Work out the finished part from the listing and answer in its coordinate system (mm). A direction names the side the tool comes from. Coordinates: 2 decimals unless noted, no trailing zeros. Loops run counter-clockwise (first coordinate to the right, second up) from the corner with the lowest first, then second, coordinate; pieces in that order, holes last. Notation, with made-up numbers: M 6.5,6 L 24.5,6 A35 ccw 24.5,41 Z; hole C 27.25,-30.75 d9. An arc over 180 degrees is marked long. Write each question's results on one line, items separated by ' | '.
```python
from build123d import *

# Parameters (mm, degrees)
EXTRUDE_THIN1_DEPTH = 80
BOSS_EXTRUDE1_REACH = 163.189
SKETCH2_W           = 20
SKETCH2_H           = 80


with BuildPart() as part:
    # Sketch1 → Extrude-Thin1 (new body)
    with BuildSketch(Plane.XY):
        with BuildLine():
            Line((0, 80), (0, 0))
            Line((0, 0), (85, 0))
            ThreePointArc((85, 0), (105.664665971, 60.876142901), (159.11809549, 96.592582629))
            Line((159.11809549, 96.592582629), (161.188647851, 88.865176019))
            ThreePointArc((161.188647851, 88.865176019), (109.643288684, 52.776567335), (93.348486101, -8))
            Line((93.348486101, -8), (-8, -8))
            Line((-8, -8), (-8, 80))
            Line((-8, 80), (0, 80))
        make_face()
    extrude(amount=EXTRUDE_THIN1_DEPTH)

    # Sketch2 → Boss-Extrude1 (add, up to next)
    with BuildSketch(Plane(origin=(0, 0, 0), x_dir=(0, 0, -1), z_dir=(1, 0, 0)), mode=Mode.PRIVATE) as boss_extrude1_sk1:
        with Locations((-40, 40)):
            Rectangle(SKETCH2_W, SKETCH2_H)
    boss_extrude1_tool1 = extrude(boss_extrude1_sk1.sketch, amount=BOSS_EXTRUDE1_REACH, mode=Mode.PRIVATE) - part.part
    add(boss_extrude1_tool1.solids().sort_by_distance((0, 40, 40))[0])


solid = part.part
```
1) Find section A-A, the plane z = 22.5. Give the vertices of the cut face in (x, y).
Check result:
outline: M -8,-8 L 93.35,-8 A92 cw 161.19,88.87 L 159.12,96.59 A100 ccw 85,0 L 0,0 L 0,80 L -8,80 Z
2) Given pin 1 Ø4 at (x, z) = (42, 55) entering from +Y; pin 2 Ø3 at (x, z) = (104, 61.5) entering from +Y; pin 3 Ø10 at (x, z) = (69.5, 30.5) entering from +Y, each flat-ended and moving along its own axis, determine where each tip first touches the part or whether it passes through.
Check result:
pin 1: y = 0 | pin 2: y = 60.66 | pin 3: y = 80
3) Straight lines are drawn through the part: probe 1 along X at (y, z) = (25, 10); probe 2 along X at (y, z) = (34, 60); probe 3 along Y at (x, z) = (83, 62). For each, find the intervals that lie inside material, in ascending order. Write a range as [from, to].
Check result:
probe 1: [-8, 0], [88.18, 96.46] | probe 2: [-8, 0], [90.96, 99.51] | probe 3: [-8, 0]
4) Find section B-B, the plane x = 66. Give the vertices of the cut face in (y, z).
Check result:
outline: M -8,0 L 0,0 L 0,30 L 80,30 L 80,50 L 0,50 L 0,80 L -8,80 Z
5) Find section C-C, the plane y = 16. Give the vertices of the cut face in (x, z), and give its area (3 significant figures).
Check result:
outline: M -8,0 L 0,0 L 0,30 L 86.29,30 L 86.29,0 L 94.4,0 L 94.4,80 L 86.29,80 L 86.29,50 L 0,50 L 0,80 L -8,80 Z | area: 3,010 mm^2
6) For a pull along X with two mould halves and no side action, classify faces 1 (the face through (42, 0, 65)), 2 (the face through (43, -8, 39)), 3 (the face through (110.16, 53.51, 39.44)) as released by +X, released by -X, zero draft, split by the parting line, or undercut.
Check result:
face 1: undercut | face 2: zero draft | face 3: released by +X
7) Which of the six approach directions +Z, -Z, +X, -X, +Y, -Y give full straight-line access (tool end or side, diameter ignored) to faces 4 (the face through (105, 60, 22)), 5 (the face through (43, 80, 39)), 6 (the face through (42, 0, 15)), 7 (the face through (48, 39, 50))?
Check result:
face 4: +Y | face 5: +Z, -Z, -X, +Y | face 6: -Z, +Y | face 7: +Z, +Y
8) Find section D-D, the plane y = 66. Give the vertices of the cut face in (x, z), and give its area (3 significant figures).
Check result:
outline: M -8,0 L 0,0 L 0,30 L 109.87,30 L 109.87,0 L 120.91,0 L 120.91,80 L 109.87,80 L 109.87,50 L 0,50 L 0,80 L -8,80 Z | area: 3,720 mm^2
